from build123d import *

# Parameters (mm, degrees)
F0_R     = 3.5
F1_DEPTH = 6.1


with BuildPart() as f1:
    # F0 (on Top) → F1 (new body)
    with BuildSketch(Plane.XY):
        Polygon((21.76044, 11.477244), (5.01044, 11.477244), (5.01044, -11.022756), (11.08544, -11.022756), (11.08544, -15.872756), (15.68544, -15.872756), (15.68544, -11.022756), (21.76044, -11.022756), align=None)
        with Locations((13.38544, 3.102244)):
            Circle(F0_R, mode=Mode.SUBTRACT)
    extrude(amount=F1_DEPTH)


solid = f1.part
For this review, take the finished solid that the model builds, in its own axes (mm). A direction names the side the tool comes from. Coordinates: 2 decimals unless noted, no trailing zeros. Loops run counter-clockwise (first coordinate to the right, second up) from the corner with the lowest first, then second, coordinate; pieces in that order, holes last. Notation, with made-up numbers: (-23, -4.5) - (-12, -4.5) arc R24 ccw to (-12, 11.5) - close; hole circle Ø1 at (-12, 34.5). An arc over 180 degrees is marked (long way). Use a Markdown table: item, result. Add a question column.
Item 1: We need section B-B (y = 3.5). Give the boundary of the cut face in (x, z).
Item 2: Mouldability with a two-part tool opening along Y and no side actions: class faces 4 (the face through (14, 11.477, 3)), 5 (the face through (21.76, 0, 3)), 6 (the face through (8, -11.023, 3)), 7 (the face through (12.627, -0.315, 3.007)) as pulls with the +Y half, pulls with the -Y half, needs draft (parallel to the pull), parting line crosses it, or undercut.
Item 3: We need section D-D (y = -13.5). Give the boundary of the cut face in (x, z), and give its area (3 significant figures).
Item 4: For line 1 (Y direction, x = 13.5, z = 1.5); line 2 (Y direction, x = 6.5, z = 2.5); line 3 (Y direction, x = 16.25, z = 1.75), list the stretches that pass through material, from the lowest coordinate up.
Item 5: We need section C-C (z = 4.5). Give the boundary of the cut face in (x, y), and give its area (3 significant figures).
Item 6: Tool access review of faces 1 (the face through (15.685, -13, 3)), 2 (the face through (5.01, 0, 3)), 3 (the face through (11.085, -13, 3)): name each direction out of +Z, -Z, +X, -X, +Y, -Y from which nothing blocks a thin tool from reaching the whole face with its end or side.
Item 7: We need section A-A (x = 10.5). Give the boundary of the cut face in (y, z), and give its area (3 significant figures).
Item 8: Insertion check: pin 1 Ø1.8 at (x, z) = (9.5, 4.5) entering from -Y. The pin has a flat end and moves straight along its axis. Give the tip position at first contact, or say it passes through.
Results list:
| question | item | result |
|---|---|---|
| 1 | outline | (5.01, 0) - (9.91, 0) - (9.91, 6.1) - (5.01, 6.1) - close; (16.86, 0) - (21.76, 0) - (21.76, 6.1) - (16.86, 6.1) - close |
| 2 | face 4 | pulls with the +Y half |
| 2 | face 5 | needs draft |
| 2 | face 6 | pulls with the -Y half |
| 2 | face 7 | undercut |
| 3 | outline | (11.09, 0) - (15.69, 0) - (15.69, 6.1) - (11.09, 6.1) - close |
| 3 | area | 28.1 mm^2 |
| 4 | line 1 | y = -15.87 to -0.4, 6.6 to 11.48 |
| 4 | line 2 | y = -11.02 to 11.48 |
| 4 | line 3 | y = -11.02 to 1.09, 5.11 to 11.48 |
| 5 | outline | (5.01, -11.02) - (11.09, -11.02) - (11.09, -15.87) - (15.69, -15.87) - (15.69, -11.02) - (21.76, -11.02) - (21.76, 11.48) - (5.01, 11.48) - close; hole circle Ø7 at (13.39, 3.1) |
| 5 | area | 361 mm^2 |
| 6 | face 1 | +Z, -Z, +X, -Y |
| 6 | face 2 | +Z, -Z, -X, +Y, -Y |
| 6 | face 3 | +Z, -Z, -X, -Y |
| 7 | outline | (-11.02, 0) - (1.12, 0) - (1.12, 6.1) - (-11.02, 6.1) - close; (5.08, 0) - (11.48, 0) - (11.48, 6.1) - (5.08, 6.1) - close |
| 7 | area | 113 mm^2 |
| 8 | pin 1 | stops at y = -11.02 |
